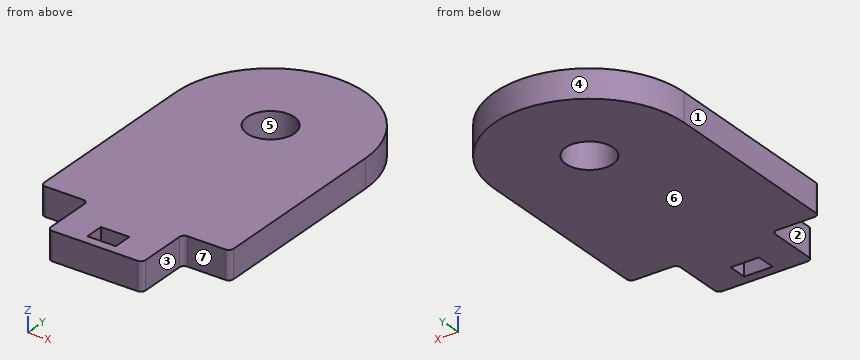
from build123d import *

# Parameters (mm, degrees)
SKETCH1_W           = 6
SKETCH1_H           = 4
BOSS_EXTRUDE1_DEPTH = 6
FILLET1_R           = 1
SKETCH2_R           = 5
CUT_EXTRUDE1_DEPTH  = 75.966659256


with BuildPart() as part:
    # Sketch1 → Boss-Extrude1 (new body)
    with BuildSketch(Plane.XY):
        with BuildLine():
            Line((-10, 0), (10, 0))
            Line((10, 0), (10, 12))
            Line((10, 12), (20, 12))
            Line((20, 12), (20, 52))
            ThreePointArc((20, 52), (0, 72), (-20, 52))
            Line((-20, 52), (-20, 12))
            Line((-20, 12), (-10, 12))
            Line((-10, 12), (-10, 0))
        make_face()
        with Locations((0, 4)):
            Rectangle(SKETCH1_W, SKETCH1_H, mode=Mode.SUBTRACT)
    extrude(amount=BOSS_EXTRUDE1_DEPTH)

    # Fillet1
    fillet1_edges = [part.edges().sort_by_distance(p)[0] for p in [
        (10, 0, 3),
        (-10, 0, 3),
        (-10, 12, 3),
        (-20, 12, 3),
        (20, 12, 3),
        (10, 12, 3),
    ]]
    fillet(fillet1_edges, radius=FILLET1_R)

    # Sketch2 → Cut-Extrude1 (cut, through all)
    with BuildSketch(Plane.XY.offset(6)):
        with Locations((0, 52)):
            Circle(SKETCH2_R)
    extrude(amount=-CUT_EXTRUDE1_DEPTH, mode=Mode.SUBTRACT)


solid = part.part
Could you check a few things on this model? Use its own coordinates, in mm. Face numbers are marked on the shaded views. A direction names the side the tool comes from. Round coordinates to 2 decimals unless told otherwise and drop trailing zeros. Order: outer loops, then holes, each group sorted by start corner. A loop starts at its lowest first (then second) coordinate and runs counter-clockwise, first axis right, second up.
Q1. Imagine slicing it at A-A, the plane x = 0. List the corners of the cut face in (y, z) for me, then the cut area to 3 significant figures.
Geometry says:
outline: (0, 0) - (2, 0) - (2, 6) - (0, 6) - close; (6, 0) - (47, 0) - (47, 6) - (6, 6) - close; (57, 0) - (72, 0) - (72, 6) - (57, 6) - close
area: 348 mm2
Q2. Please list where these lines run through material, in increasing order: probe 1 along Y at (x, z) = (0, 4.1); probe 2 along X at (y, z) = (7.5, 4.7); probe 3 along X at (y, z) = (56, 0.4).
Geometry says:
probe 1: y = 0 to 2, 6 to 47, 57 to 72
probe 2: x = -10 to 10
probe 3: x = -19.6 to -3, 3 to 19.6
Q3. I'm going to push flat-ended pins straight in: P1, Ø3, axis at x = 1, z = 2.5, coming from the +Y side; P2, Ø1.2, axis at y = 3, z = 4, coming from the -X side; P3, Ø3, axis at x = -13.5, z = 4, coming from the +Y side. Where does each tip first touch, or does it pass through?
Geometry says:
P1: stops at y = 72
P2: stops at x = -10
P3: stops at y = 68
Q4. Imagine slicing it at C-C, the plane y = 65. List the corners of the cut face in (x, z) for me.
Geometry says:
outline: (-15.2, 0) - (15.2, 0) - (15.2, 6) - (-15.2, 6) - close
Q5. Imagine slicing it at B-B, the plane z = 1.35. List the corners of the cut face in (x, y) for me.
Geometry says:
outline: (-20, 13) arc R1 ccw to (-19, 12) - (-11, 12) arc R1 cw to (-10, 11) - (-10, 1) arc R1 ccw to (-9, 0) - (9, 0) arc R1 ccw to (10, 1) - (10, 11) arc R1 cw to (11, 12) - (19, 12) arc R1 ccw to (20, 13) - (20, 52) arc R20 ccw to (-20, 52) - close; hole circle Ø10 at (0, 52); hole (-3, 2) - (3, 2) - (3, 6) - (-3, 6) - close
Q6. Thinking about a two-plate mould opening in Y: for the marked faces 4, 5, 6 and 7, which applies, released by +Y, released by -Y, zero draft, split by the parting line, or undercut?
Geometry says:
face 4: released by +Y
face 5: undercut
face 6: zero draft
face 7: released by -Y
Q7. Which directions (+Z, -Z, +X, -X, +Y, -Y) give clear straight access to the entire face, cutting with the end or side of a thin tool? Please do the marked faces 1, 2 and 3.
Geometry says:
face 1: +Z, -Z, -X, +Y, -Y
face 2: +Z, -Z, -X, -Y
face 3: +Z, -Z, +X, -Y
Q8. Imagine slicing it at D-D, the plane x = 14.5. List the corners of the cut face in (y, z) for me, then the cut area to 3 significant figures.
Geometry says:
outline: (12, 0) - (65.77, 0) - (65.77, 6) - (12, 6) - close
area: 323 mm2
